from build123d import *

# Parameters (mm, degrees)
SKETCH2_R = 0.65


with BuildPart() as part:
    # Sweep1: sweep along a path in Sketch1
    with BuildLine(Plane.XY) as sweep1_path:
        Line((85, 0), (0, 0))
        ThreePointArc((0, 0), (-1.414213562, 0.585786438), (-2, 2))
        Line((-2, 2), (-2, 5))
        ThreePointArc((-2, 5), (-2.585786438, 6.414213562), (-4, 7))
        Line((-4, 7), (-7, 7))
    # Sketch2 → Sweep1 (sweep)
    with BuildSketch(Plane(origin=(85, 0, 0), x_dir=(0, 0, -1), z_dir=(1, 0, 0))):
        Circle(SKETCH2_R)
    sweep(path=sweep1_path.line)


solid = part.part
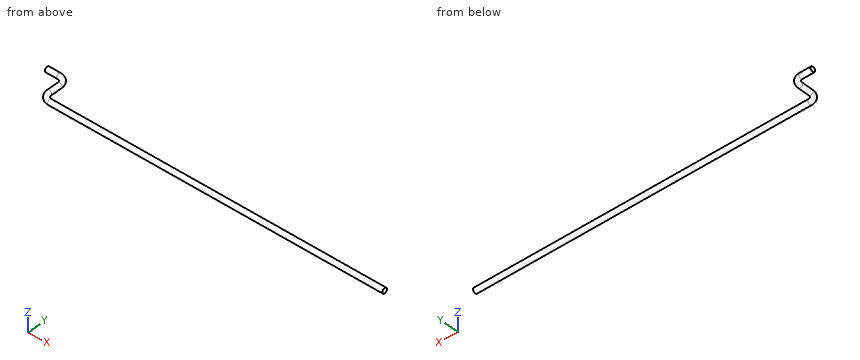
For this review, take the finished solid that the model builds, in its own axes (mm). Round coordinates to 2 decimals unless told otherwise and drop trailing zeros. Order: outer loops, then holes, each group sorted by start corner. A loop starts at its lowest first (then second) coordinate and runs counter-clockwise, first axis right, second up. Notation, with made-up numbers: (63, 62) -> (96, 62) arc R33 cw to (96, 91) -> close; hole circle Ø5 at (46, 88). An arc over 180 degrees is marked (long way). Put each result on its own line as item: value.
Q1. Add section B-B on y = 3. Write out the cut boundary in (x, z).
Check result:
outline: circle Ø1.3 at (-2, 0)
Q2. For probe 1 along Y at (x, z) = (65, 0); probe 2 along X at (y, z) = (7.25, -0.15); probe 3 along Y at (x, z) = (28.5, 0.4), list the stretches that pass through material, from the lowest coordinate up. Write a range as [from, to].
Check result:
probe 1: [-0.65, 0.65]
probe 2: [-7, -2.63]
probe 3: [-0.51, 0.51]
Q3. Add section A-A on z = 0. Write out the cut boundary in (x, y).
Check result:
outline: (-7, 6.35) -> (-4, 6.35) arc R1.35 cw to (-2.65, 5) -> (-2.65, 2) arc R2.65 ccw to (0, -0.65) -> (85, -0.65) -> (85, 0.65) -> (0, 0.65) arc R1.35 cw to (-1.35, 2) -> (-1.35, 5) arc R2.65 ccw to (-4, 7.65) -> (-7, 7.65) -> close
Q4. Add section C-C on x = 68.5. Write out the cut boundary in (y, z).
Check result:
outline: circle Ø1.3 at (0, 0)
